Geometry: final body of the model. Coordinates: model frame, mm. A direction names the side the tool comes from. Give positions to 0.01 mm unless a question says otherwise; leave off trailing zeros. Write each loop counter-clockwise with the first axis right and the second up, starting at its lowest first coordinate (ties: lowest second). Pieces come first, ordered by that corner, then holes. Notation, with made-up numbers: M -32,80 L 23,80 A18 ccw 23,84 Z; hole C 60,-35.75 d1. An arc over 180 degrees is marked long. Use a Markdown table: item, result. Add a question column.
(1) Material intervals for L1, parallel to Y at x = 36.5, z = 0.65; L2, parallel to Y at x = 12, z = 18; L3, parallel to X at y = -13.5, z = 10.5, sorted ascending.
(2) Cut plane D-D (y = -27). Output: boundary loops of the cut face in (x, z), plus the area to 3 significant figures.
(3) Cut plane A-A (z = 17.5). Output: boundary loops of the cut face in (x, y).
(4) Pin query (flat end, axial travel): pin 1 Ø1.5 at (x, z) = (0.5, 3.5) entering from +Y; pin 2 Ø1 at (x, z) = (2.5, 8) entering from -Y; pin 3 Ø0.8 at (x, z) = (38, 0.5) entering from +Y. Return the tip coordinate at first contact, or that it passes through.
(5) Cut plane B-B (x = -36.5). Output: boundary loops of the cut face in (y, z), plus the area to 3 significant figures.
(6) Cut plane C-C (z = 6). State how many separate pieces and enclosed holes the cut face has, plus the area to 3 significant figures.
(7) Draft query along Y for faces 6 (the flat face through (0, -36, 11)), 7 (the cylindrical face through (-35.462, 28.996, 0.493)), 8 (the flat face through (-17.5, 0, 16)). Return one class per face: released by +Y, released by -Y, zero draft, split by the parting line, or undercut.
(8) Reachability of faces 1 (the flat face through (-11.5, 27, 11)), 2 (the flat face through (0, -16, 9)), 3 (the flat face through (-27.5, 0, 6)), 4 (the flat face through (-12.5, -27, 11)), 5 (the flat face through (12.5, -27, 11)) from +Z, -Z, +X, -X, +Y, -Y: full face, straight path, thin tool, end or side. Return the list, or none.
Autodesk Inventor part; units mm, degrees
ref_plane "YZ Plane" through (0, 0, 0) normal (1, 0, 0) x (0, 1, 0)
ref_plane "XZ Plane" through (0, 0, 0) normal (0, 1, 0) x (-1, 0, 0)
ref_plane "XY Plane" through (0, 0, 0) normal (0, 0, 1) x (1, 0, 0)
sketch "Sketch1" plane through (0, 0, 0) normal (0, 0, 1) x (1, 0, 0)
  line L0 (-41.5, 50) -> (41.5, 50)
  line L1 (41.5, 50) -> (41.5, -50)
  line L2 (41.5, -50) -> (-41.5, -50)
  line L3 (-41.5, -50) -> (-41.5, 50)
  line L4 (31.5, 40) -> (-31.5, 40)
  line L5 (-31.5, 40) -> (-31.5, -40)
  line L6 (-31.5, -40) -> (31.5, -40)
  line L7 (31.5, -40) -> (31.5, 40)
  line L8 (-41.5, -45) -> (41.5, -45) construction
  line L9 (0, 71.7466) -> (0, -78.0681) construction
  line L10 (-60.2597, 0) -> (74.2823, 0) construction
  line L11 (-36.5, 50) -> (-36.5, -50) construction
  circle A0 centre (-36.5, -27) radius 2.25
  line L12 (-41.5, 45) -> (41.5, 45) construction
  circle A1 centre (-36.5, 45) radius 2.25
  circle A2 centre (-36.5, -45) radius 2.25
  circle A3 centre (-36.5, 27) radius 2.25
  circle A4 centre (-25, -45) radius 2.25
  circle A5 centre (25, -45) radius 2.25
  line L13 (30, 50) -> (30, -50) construction
  line L14 (-30, 50) -> (-30, -50) construction
  line L15 (-31, -38) -> (31, -38)
  line L16 (31, -38) -> (31, -52)
  line L17 (31, -52) -> (-31, -52)
  line L18 (-31, -52) -> (-31, -38)
  line L19 (-31.5, -40) -> (-16.5, -40)
  line L20 (-16.5, -40) -> (-16.5, -20)
  line L21 (-16.5, -20) -> (-31.5, -20)
  line L22 (-31.5, -20) -> (-31.5, -40)
  line L23 (-26.5, -26) -> (-21.5, -26) construction
  line L24 (-26.5, -27.5) -> (-21.5, -27.5)
  line L25 (-21.5, -24.5) -> (-26.5, -24.5)
  arc A6 (-26.5, -24.5) -> (-26.5, -27.5) centre (-26.5, -26) ccw
  arc A7 (-21.5, -27.5) -> (-21.5, -24.5) centre (-21.5, -26) ccw
  line L26 (-26.5, -34) -> (-21.5, -34) construction
  line L27 (-26.5, -35.5) -> (-21.5, -35.5)
  line L28 (-21.5, -32.5) -> (-26.5, -32.5)
  arc A8 (-26.5, -32.5) -> (-26.5, -35.5) centre (-26.5, -34) ccw
  arc A9 (-21.5, -35.5) -> (-21.5, -32.5) centre (-21.5, -34) ccw
  point P0 (0, 0)
  point P1 (0, 50)
  point P2 (41.5, 0)
  point P3 (0, 45)
  point P4 (-24, -26)
  point P5 (-24, -20)
  point P6 (-16.5, -30)
  point P7 (-24, -34)
  dimension "d0" = 83
  dimension "d1" = 100
  dimension "d5" = 5
  dimension "d6" = 5
  dimension "d9" = 5
  dimension "d12" = 4.5
  dimension "d17" = 5
  dimension "d41" = 4.5
  dimension "d42" = 4.5
  dimension "d87" = 4.5
  dimension "d89" = 4.5
  dimension "d90" = 4.5
  dimension "d91" = 30
  dimension "d92" = 30
  dimension "d93" = 5
  dimension "d94" = 5
  dimension "d97" = 1
  dimension "d98" = 2
  dimension "d99" = 2
  dimension "d100" = 1
  dimension "d103" = 15
  dimension "d104" = 20
  dimension "d105" = 5
  dimension "d106" = 3
  dimension "d109" = 5
  dimension "d110" = 3
  dimension "d112" = 6
  dimension "d113" = 6
  dimension "d141" = 27
  dimension "d142" = 27
sketch "Sketch4" plane through (0, 0, 0) normal (0, 0, 1) x (1, 0, 0)
  circle A0 centre (-36.5, 27) radius 2.25
  circle A1 centre (-36.5, -27) radius 2.25
  line L0 (-31.5, 40) -> (-31.5, -40)
  line L1 (-41.5, -50) -> (-41.5, 50)
  line L2 (-41.5, -32.25) -> (-31.5, -32.25)
  line L3 (-31.5, -32.25) -> (-31.5, 32.25)
  line L4 (-31.5, 32.25) -> (-41.5, 32.25)
  line L5 (-41.5, 32.25) -> (-41.5, -32.25)
  line L6 (31.5, -40) -> (31.5, 40)
  line L7 (41.5, 50) -> (41.5, -50)
  line L8 (-31.5, -18) -> (31.5, -18)
  line L9 (31.5, -18) -> (31.5, 0)
  line L10 (31.5, 0) -> (-31.5, 0)
  line L11 (-31.5, 0) -> (-31.5, -18)
  line L12 (-16.5, -20) -> (-31.5, -20)
  line L13 (-31.5, -40) -> (31.5, -40)
  line L14 (-16.5, -40) -> (-16.5, -20)
  line L15 (-14.5, -18) -> (0, -18)
  line L16 (0, -18) -> (0, -38)
  line L17 (0, -38) -> (-14.5, -38)
  line L18 (-14.5, -38) -> (-14.5, -18)
  point P0 (0, 0)
  point P1 (0, 0)
  dimension "d116" = 3
  dimension "d117" = 3
  dimension "d118" = 2
  dimension "d130" = 2
  dimension "d131" = 2
extrude "Extrusion11" add sketch "Sketch4" along normal blind 1 contours L0 L2 L1 L4
extrude "Extrusion12" add sketch "Sketch4" along normal blind 1 contours L10 L6 L8 L0
mirror "Mirror4" about plane through (0, 0, 0) normal (0, 1, 0) of "Extrusion12"
mirror "Mirror5" about plane through (0, 0, 0) normal (1, 0, 0) of "Extrusion11"
sketch "Sketch6" plane through (0, 0, 1) normal (0, 0, 1) x (1, 0, 0)
  line L0 (-17.5, 16) -> (17.5, 16)
  line L1 (17.5, 16) -> (17.5, -16)
  line L2 (17.5, -16) -> (-17.5, -16)
  line L3 (-17.5, -16) -> (-17.5, 16)
  line L4 (16.5, 15) -> (-16.5, 15)
  line L5 (-16.5, 15) -> (-16.5, -15)
  line L6 (-16.5, -15) -> (16.5, -15)
  line L7 (16.5, -15) -> (16.5, 15)
  circle A0 centre (36.5, 27) radius 2.25
  circle A1 centre (36.5, -27) radius 2.25
  circle A2 centre (-36.5, -27) radius 2.25
  circle A3 centre (-36.5, 27) radius 2.25
  line L8 (-41.5, -32.25) -> (-31.5, -32.25)
  line L9 (-31.5, -32.25) -> (-31.5, -18)
  line L10 (-31.5, -18) -> (31.5, -18)
  line L11 (31.5, -32.25) -> (31.5, -18)
  line L12 (41.5, -32.25) -> (31.5, -32.25)
  line L13 (41.5, 32.25) -> (41.5, -32.25)
  line L14 (31.5, 32.25) -> (41.5, 32.25)
  line L15 (31.5, 18) -> (31.5, 32.25)
  line L16 (-31.5, 18) -> (31.5, 18)
  line L17 (-31.5, 18) -> (-31.5, 32.25)
  line L18 (-31.5, 32.25) -> (-41.5, 32.25)
  line L19 (-41.5, 32.25) -> (-41.5, -32.25)
  line L20 (-27.5, 16) -> (-17.5, 16)
  line L21 (-17.5, 16) -> (-17.5, -16)
  line L22 (-17.5, -16) -> (-27.5, -16)
  line L23 (-27.5, -16) -> (-27.5, 16)
  line L24 (-18.5, 15) -> (-26.5, 15)
  line L25 (-26.5, 15) -> (-26.5, -15)
  line L26 (-26.5, -15) -> (-18.5, -15)
  line L27 (-18.5, -15) -> (-18.5, 15)
  point P0 (0, 0)
  point P1 (0, 16)
  dimension "d123" = 1
  dimension "d124" = 2
  dimension "d126" = 2
  dimension "d143" = 14
  dimension "d144" = 2
  dimension "d145" = 2
  dimension "d146" = 1
  dimension "d147" = 10
extrude "Extrusion13" add sketch "Sketch6" along normal blind 20 contours L0 L1 L2 L3
extrude "Extrusion14" add sketch "Sketch4" along normal blind 1 contours L8 L16 L17 L18
mirror "Mirror6" about plane through (0, 0, 0) normal (1, 0, 0) of "Extrusion14"
mirror "Mirror7" about plane through (0, 0, 0) normal (0, 1, 0) of "Extrusion14", "Mirror6"
sketch "Sketch7" plane through (0, 0, 1) normal (0, 0, 1) x (1, 0, 0)
  line L0 (-41.5, -32.25) -> (-31.5, -32.25)
  line L1 (-31.5, -32.25) -> (-31.5, -18)
  line L2 (-31.5, -18) -> (-14.5, -18)
  line L3 (-14.5, -18) -> (-14.5, -38)
  line L4 (-14.5, -38) -> (14.5, -38)
  line L5 (14.5, -18) -> (14.5, -38)
  line L6 (14.5, -18) -> (31.5, -18)
  line L7 (31.5, -32.25) -> (31.5, -18)
  line L8 (41.5, -32.25) -> (31.5, -32.25)
  line L9 (41.5, 32.25) -> (41.5, -32.25)
  line L10 (31.5, 32.25) -> (41.5, 32.25)
  line L11 (31.5, 18) -> (31.5, 32.25)
  line L12 (14.5, 18) -> (31.5, 18)
  line L13 (14.5, 18) -> (14.5, 38)
  line L14 (14.5, 38) -> (-14.5, 38)
  line L15 (-14.5, 18) -> (-14.5, 38)
  line L16 (-31.5, 18) -> (-14.5, 18)
  line L17 (-31.5, 18) -> (-31.5, 32.25)
  line L18 (-31.5, 32.25) -> (-41.5, 32.25)
  line L19 (-41.5, 32.25) -> (-41.5, -32.25)
  circle A0 centre (-36.5, 27) radius 2.25
  circle A1 centre (-36.5, -27) radius 2.25
  circle A2 centre (36.5, -27) radius 2.25
  circle A3 centre (36.5, 27) radius 2.25
  line L20 (17.5, 16) -> (17.5, -16)
  line L21 (17.5, -16) -> (-17.5, -16)
  line L22 (-17.5, -16) -> (-17.5, 16)
  line L23 (-17.5, 16) -> (17.5, 16)
  line L24 (-12.5, 36) -> (12.5, 36)
  line L25 (12.5, 36) -> (12.5, 18)
  line L26 (12.5, 18) -> (-12.5, 18)
  line L27 (-12.5, 18) -> (-12.5, 36)
  line L28 (11.5, 35) -> (-11.5, 35)
  line L29 (-11.5, 35) -> (-11.5, 19)
  line L30 (-11.5, 19) -> (11.5, 19)
  line L31 (11.5, 19) -> (11.5, 35)
  point P0 (0, 0)
  dimension "d134" = 1
  dimension "d135" = 2
  dimension "d136" = 2
  dimension "d137" = 2
  dimension "d138" = 2
extrude "Extrusion15" add sketch "Sketch7" along normal blind 20 contours L24 L25 L26 L27
mirror "Mirror8" about plane through (0, 0, 0) normal (0, 1, 0) of "Extrusion15"
extrude "Extrusion16" add sketch "Sketch6" along normal blind 10 contours L3 L22 L23 L20
mirror "Mirror9" about plane through (0, 0, 0) normal (1, 0, 0) of "Extrusion16"
equation "\"d12\" = screw"
equation "\"d41\" = screw"
equation "\"d42\" = screw"
equation "\"d87\" = screw"
equation "\"d89\" = screw"
equation "\"d90\" = screw"
properties part number "Side" material "PC/ABS Plastic"
Answer list:
| question | item | result |
|---|---|---|
| 1 | L1 | -32.25 to -29.25, -24.75 to 24.75, 29.25 to 32.25 |
| 1 | L2 | -36 to -18, -16 to -15, 15 to 16, 18 to 36 |
| 1 | L3 | -27.5 to -26.5, -18.5 to -16.5, 16.5 to 18.5, 26.5 to 27.5 |
| 2 | outline | M -41.5,0 L -38.75,0 L -38.75,1 L -41.5,1 Z; M -34.25,0 L -31.5,0 L -31.5,1 L -34.25,1 Z; M -14.5,0 L 14.5,0 L 14.5,1 L 12.5,1 L 12.5,21 L 11.5,21 L 11.5,1 L -11.5,1 L -11.5,21 L -12.5,21 L -12.5,1 L -14.5,1 Z; M 31.5,0 L 34.25,0 L 34.25,1 L 31.5,1 Z; M 38.75,0 L 41.5,0 L 41.5,1 L 38.75,1 Z |
| 2 | area | 80.0 mm² |
| 3 | outline | M -17.5,-16 L 17.5,-16 L 17.5,16 L -17.5,16 Z; M -12.5,-36 L 12.5,-36 L 12.5,-18 L -12.5,-18 Z; M -12.5,18 L 12.5,18 L 12.5,36 L -12.5,36 Z; hole M -16.5,-15 L 16.5,-15 L 16.5,15 L -16.5,15 Z; hole M -11.5,-35 L 11.5,-35 L 11.5,-19 L -11.5,-19 Z; hole M -11.5,19 L 11.5,19 L 11.5,35 L -11.5,35 Z |
| 4 | pin 1 | y = 36 |
| 4 | pin 2 | y = -36 |
| 4 | pin 3 | y = 32.25 |
| 5 | outline | M -32.25,0 L -29.25,0 L -29.25,1 L -32.25,1 Z; M -24.75,0 L 24.75,0 L 24.75,1 L -24.75,1 Z; M 29.25,0 L 32.25,0 L 32.25,1 L 29.25,1 Z |
| 5 | area | 55.5 mm² |
| 6 | separate pieces | 3 |
| 6 | enclosed holes | 5 |
| 6 | area | 454 mm² |
| 7 | face 6 | released by -Y |
| 7 | face 7 | undercut |
| 7 | face 8 | zero draft |
| 8 | face 1 | +Z |
| 8 | face 2 | +Z, +X, -X |
| 8 | face 3 | +Z, -X, +Y, -Y |
| 8 | face 4 | +Z, -X, -Y |
| 8 | face 5 | +Z, +X, -Y |
